from build123d import *

# Parameters (mm, degrees)
CUT_EXTRUDE1_DEPTH = 15
SKETCH4_R          = 2.9
CUT_EXTRUDE2_DEPTH = 17.425
SKETCH5_R          = 3
CUT_EXTRUDE3_DEPTH = 180


with BuildPart() as part:
    # Sketch2 → Revolve1 (revolve)
    with BuildSketch(Plane(origin=(0, 0, 0), x_dir=(0, 0, -1), z_dir=(1, 0, 0))):
        Polygon((116.173333333, 10.525), (116.173333333, 8), (131.173333333, 8), (131.173333333, 0), (-102.826666667, 0), (-102.826666667, 8), (-87.826666667, 8), (-87.826666667, 10.525), (-77.826666667, 10.525), (-77.826666667, 10), (106.173333333, 10), (106.173333333, 10.525), align=None)
    revolve(axis=Axis((0, 0, -131.173333333), (0, 0, 1)))

    # Sketch3 → Cut-Extrude1 (cut)
    with BuildSketch(Plane.XY.offset(102.826666667)):
        with BuildLine():
            Line((-5.9, 5.402777064), (-5.9, -5.402777064))
            ThreePointArc((-5.9, -5.402777064), (-8, 0), (-5.9, 5.402777064))
        make_face()
        with BuildLine():
            Line((5.9, -5.402777064), (5.9, 5.402777064))
            ThreePointArc((5.9, 5.402777064), (8, 0), (5.9, -5.402777064))
        make_face()
    extrude(amount=-CUT_EXTRUDE1_DEPTH, mode=Mode.SUBTRACT)

    # Sketch4 → Cut-Extrude2 (cut, through all)
    with BuildSketch(Plane(origin=(5.9, 0, 0), x_dir=(0, 0, -1), z_dir=(1, 0, 0))):
        with Locations(Location((-95.926666667, 0, 0), (0, 0, 90))):  # turned: the seam where the file's is
            Circle(SKETCH4_R)
    extrude(amount=-CUT_EXTRUDE2_DEPTH, mode=Mode.SUBTRACT)

    # Sketch5 → Cut-Extrude3 (cut)
    with BuildSketch(Plane(origin=(0, 0, -131.173333333), x_dir=(-1, 0, 0), z_dir=(0, 0, -1))):
        with Locations(Location((0, 0, 0), (0, 0, 90))):  # turned: the seam where the file's is
            Circle(SKETCH5_R)
    extrude(amount=-CUT_EXTRUDE3_DEPTH, mode=Mode.SUBTRACT)


solid = part.part
Input: part model. Units: mm. Frame: model coordinates. A direction names the side the tool comes from. Coordinates: 2 decimals unless noted, no trailing zeros. Loops run counter-clockwise (first coordinate to the right, second up) from the corner with the lowest first, then second, coordinate; pieces in that order, holes last.
(1) Material intervals for probe 1 along X at (y, z) = (-0.5, -105); probe 2 along Z at (x, y) = (3.5, -9.5), sorted ascending.
(2) Section A-A on y = 0. Return the cut outline in (x, z) (3 decimals), then the cut area to 3 significant figures.
(3) Section C-C on z = -72. Return the cut outline in (x, y).
(4) Section B-B on x = 0. Return the cut outline in (y, z) (3 decimals), then the cut area to 3 significant figures.
(5) Set-up query: faces 4 (the face through (7, 0, 87.827)), 5 (the face through (0, -8, 95)), 6 (the face through (5.9, -2.5, 93.8)). Return all of +Z, -Z, +X, -X, +Y, -Y with unobstructed straight access to the full face (end or side cutting, diameter ignored); none if empty.
(6) Pull-direction query (Y, two-part tool) for faces 1 (the face through (0.1, -0.4, 98.8)), 2 (the face through (-3.16, 10.04, 82.76)), 3 (the face through (-5.9, 2.5, 93.8)); classes: released by +Y, released by -Y, zero draft, split by the parting line, or undercut.
(7) Section D-D on z = 82. Return the cut outline in (x, y) (3 decimals), then the cut area to 3 significant figures.
(8) First-contact query: pin 1 Ø2 at (x, y) = (1.5, -2) entering from -Z; pin 2 Ø1.8 at (x, y) = (-0.5, -1) entering from -Z; pin 3 Ø1 at (y, z) = (-1, 47.5) entering from -X; pin 4 Ø3 at (y, z) = (2.5, 97) entering from -X. Flat tips, straight axial feed; report the tip coordinate or a pass-through.
Data:
1. probe 1: x = -9.99 to -2.96, 2.96 to 9.99
1. probe 2: z = -116.17 to -106.17, 77.83 to 87.83
2. outline: (-10.525, -116.173) - (-8, -116.173) - (-8, -131.173) - (-3, -131.173) - (-3, 48.827) - (3, 48.827) - (3, -131.173) - (8, -131.173) - (8, -116.173) - (10.525, -116.173) - (10.525, -106.173) - (10, -106.173) - (10, 77.827) - (10.525, 77.827) - (10.525, 87.827) - (5.9, 87.827) - (5.9, 93.027) - (-5.9, 93.027) - (-5.9, 87.827) - (-10.525, 87.827) - (-10.525, 77.827) - (-10, 77.827) - (-10, -106.173) - (-10.525, -106.173) - close; (-5.9, 98.827) - (5.9, 98.827) - (5.9, 102.827) - (-5.9, 102.827) - close
2. area: 3,370 mm2
3. outline: circle Ø20 at (0, 0); hole circle Ø6 at (0, 0)
4. outline: (-10.525, -116.173) - (-8, -116.173) - (-8, -131.173) - (-3, -131.173) - (-3, 48.827) - (3, 48.827) - (3, -131.173) - (8, -131.173) - (8, -116.173) - (10.525, -116.173) - (10.525, -106.173) - (10, -106.173) - (10, 77.827) - (10.525, 77.827) - (10.525, 87.827) - (8, 87.827) - (8, 102.827) - (-8, 102.827) - (-8, 87.827) - (-10.525, 87.827) - (-10.525, 77.827) - (-10, 77.827) - (-10, -106.173) - (-10.525, -106.173) - close; hole circle Ø5.8 at (0, 95.927)
4. area: 3,470 mm2
5. face 4: +Z
5. face 5: +Z, -Y
5. face 6: +Z, +X, +Y, -Y
6. face 1: undercut
6. face 2: split by the parting line
6. face 3: zero draft
7. outline: circle Ø21.05 at (0, 0)
7. area: 348 mm2
8. pin 1: stops at z = -131.17
8. pin 2: stops at z = 48.83
8. pin 3: stops at x = -9.99
8. pin 4: stops at x = -5.9
